Input: part model. Units: mm. Frame: model coordinates. A direction names the side the tool comes from. Coordinates: 2 decimals unless noted, no trailing zeros. Order: outer loops, then holes, each group sorted by start corner. A loop starts at its lowest first (then second) coordinate and runs counter-clockwise, first axis right, second up. Notation, with made-up numbers: (-3, 12) - (26, 12) arc R14 cw to (26, 21) - close; hole circle Ø6 at (9.25, -34). An arc over 180 degrees is marked (long way). Use a Markdown table: item, result. Add a question column.
from build123d import *

# Parameters (mm, degrees)
SKETCH1_R          = 2.65
SKETCH1_R_2        = 1.6
EXTRUDE1_DEPTH     = 3
SKETCH2_R          = 20
CUT_EXTRUDE1_DEPTH = 3


with BuildPart() as part:
    # Sketch1 → Extrude1 (new body)
    with BuildSketch(Plane.XY):
        Polygon((-33.99999989, 52.265), (-33.99999989, 37.844541986), (-18.99999989, 10.293251102), (-18.99999989, -7.768251102), (-33.99999989, -35.319541986), (-33.99999989, -49.74), (-2, -49.74), (22.501120576, -4.7375), (22.501120576, 7.2625), (-2, 52.265), align=None)
        with Locations((-27.99999989, 44.265)):
            Circle(SKETCH1_R, mode=Mode.SUBTRACT)
        with Locations((-8, 44.262899898)):
            Circle(SKETCH1_R, mode=Mode.SUBTRACT)
        with Locations((-27.99999989, -41.737899898)):
            Circle(SKETCH1_R, mode=Mode.SUBTRACT)
        with Locations((-8, -41.74)):
            Circle(SKETCH1_R, mode=Mode.SUBTRACT)
        with Locations((0.071120582, 11.2625)):
            Circle(SKETCH1_R_2, mode=Mode.SUBTRACT)
        with Locations((13.571120582, 1.2625)):
            Circle(SKETCH1_R_2, mode=Mode.SUBTRACT)
        with Locations((0.071120582, -8.7375)):
            Circle(SKETCH1_R_2, mode=Mode.SUBTRACT)
        with BuildLine():
            Line((7.571120582, -2.2375), (7.571120582, 4.7625))
            ThreePointArc((7.571120582, 4.7625), (7.131780753, 5.823160172), (6.071120582, 6.2625))
            Line((6.071120582, 6.2625), (-12.928879418, 6.2625))
            ThreePointArc((-12.928879418, 6.2625), (-13.98953959, 5.823160172), (-14.428879418, 4.7625))
            Line((-14.428879418, 4.7625), (-14.428879418, -2.2375))
            ThreePointArc((-14.428879418, -2.2375), (-13.98953959, -3.298160172), (-12.928879418, -3.7375))
            Line((-12.928879418, -3.7375), (6.071120582, -3.7375))
            ThreePointArc((6.071120582, -3.7375), (7.131780753, -3.298160172), (7.571120582, -2.2375))
        make_face(mode=Mode.SUBTRACT)
    extrude(amount=EXTRUDE1_DEPTH)

    # Sketch2 → Cut-Extrude1 (cut)
    with BuildSketch(Plane.XY.offset(3)):
        with Locations((22.501120582, 31.14)):
            Circle(SKETCH2_R)
        with Locations((22.501120582, -28.86)):
            Circle(SKETCH2_R)
    extrude(amount=-CUT_EXTRUDE1_DEPTH, mode=Mode.SUBTRACT)


solid = part.part
1) Cut plane A-A (x = -8). Return the cut outline in (y, z) (1 decimal), and give its area (3 significant figures).
2) Cut plane D-D (y = -23.5). Return the cut outline in (x, z), and give its area (3 significant figures).
3) Reachability of faces 4 (the flat face through (-4, -3.738, 1)), 5 (the flat face through (1.357, 46.099, 1.479)), 6 (the flat face through (-19, 1, 1)) from +Z, -Z, +X, -X, +Y, -Y: full face, straight path, thin tool, end or side. Return the list, or none.
4) Contact query for flat-ended pins moving along their axis: P1, Ø1.5, axis at y = -24, z = 2.5, coming from the +X side; P2, Ø1.5, axis at x = 0.5, z = 1, coming from the +Y side; P3, Ø1.5, axis at y = 3, z = 1, coming from the -X side. Output: stop coordinate, or through.
5) Cut plane B-B (z = 0.9). State how many separate pieces and enclosed holes the cut face has, and give its area (3 significant figures).
6) Cut plane C-C (x = -23). Return the cut outline in (y, z) (3 decimals), and give its area (3 significant figures).
7) Material intervals for L1, parallel to Y at x = -8, z = 1.15 (1 decimal); L2, parallel to Y at x = -12, z = 0.6 (1 decimal); L3, parallel to Y at x = -6, z = 1.9 (1 decimal), sorted ascending.
8) Pull-direction query (Y, two-part tool) for faces 1 (the flat face through (-18, 52.265, 1)), 2 (the flat face through (-18, -49.74, 1)), 3 (the cylindrical face through (5.065, -19.062, 1.521)); classes: pulls with the +Y half, pulls with the -Y half, needs draft (parallel to the pull), parting line crosses it, or undercut.
Computed:
| question | item | result |
|---|---|---|
| 1 | outline | (-49.7, 0) - (-44.4, 0) - (-44.4, 3) - (-49.7, 3) - close; (-39.1, 0) - (-3.7, 0) - (-3.7, 3) - (-39.1, 3) - close; (6.3, 0) - (41.6, 0) - (41.6, 3) - (6.3, 3) - close; (46.9, 0) - (52.3, 0) - (52.3, 3) - (46.9, 3) - close |
| 1 | area | 244 mm2 |
| 2 | outline | (-27.56, 0) - (3.23, 0) - (3.23, 3) - (-27.56, 3) - close |
| 2 | area | 92.4 mm2 |
| 3 | face 4 | +Z, -Z |
| 3 | face 5 | +Z, -Z, +X, +Y |
| 3 | face 6 | +Z, -Z, -X |
| 4 | P1 | stops at x = 3.3 |
| 4 | P2 | stops at y = 49.05 |
| 4 | P3 | stops at x = -19 |
| 5 | separate pieces | 1 |
| 5 | enclosed holes | 8 |
| 5 | area | 3,250 mm2 |
| 6 | outline | (-49.74, 0) - (-15.115, 0) - (-15.115, 3) - (-49.74, 3) - close; (17.64, 0) - (52.265, 0) - (52.265, 3) - (17.64, 3) - close |
| 6 | area | 208 mm2 |
| 7 | L1 | y = -49.7 to -44.4, -39.1 to -3.7, 6.3 to 41.6, 46.9 to 52.3 |
| 7 | L2 | y = -49.7 to -3.7, 6.3 to 52.3 |
| 7 | L3 | y = -49.7 to -43.5, -40 to -3.7, 6.3 to 42.5, 46 to 52.3 |
| 8 | face 1 | pulls with the +Y half |
| 8 | face 2 | pulls with the -Y half |
| 8 | face 3 | undercut |
